The model under review builds one solid part; all positions refer to its coordinate system, in mm. A direction names the side the tool comes from. Give positions to 0.01 mm unless a question says otherwise; leave off trailing zeros. Loops run counter-clockwise (first coordinate to the right, second up) from the corner with the lowest first, then second, coordinate; pieces in that order, holes last. Notation, with made-up numbers: (-33.75, -25) - (-16.75, -25) arc R25 cw to (-16.75, -4) - close; hole circle Ø3 at (15, 37.25). An arc over 180 degrees is marked (long way). Return JSON: item names as keys, results as strings. Group by question number.
from build123d import *

# Parameters (mm, degrees)
SKETCH1_W                   = 12.7
SKETCH1_H                   = 483
BOSS_EXTRUDE1_DEPTH         = 3.175
EDGE_FLANGE1_DEPTH          = 12.7
TAP_DRILL_FOR_M4X0_7_TAP1_D = 3.3


# Sheet-metal steps are written as plain solids
with BuildPart() as part:
    # Sketch1 → Boss-Extrude1 (new body)
    with BuildSketch(Plane.XY):
        with Locations((6.35, 241.5)):
            Rectangle(SKETCH1_W, SKETCH1_H)
    extrude(amount=BOSS_EXTRUDE1_DEPTH)

    # Edge-Flange1 section (across the edge) → Edge-Flange1 (add)
    with BuildSketch(Plane(origin=(0, 493.5, 0), x_dir=(0, -1, 0), z_dir=(1, 0, 0))):
        with BuildLine():
            Line((-3.175, 10.5), (-3.175, 52.825))
            Line((-3.175, 52.825), (0, 52.825))
            Line((0, 52.825), (0, 10.5))
            ThreePointArc((0, 10.5), (3.075378798, 3.075378798), (10.5, 0))
            Line((10.5, 0), (10.5, -3.175))
            ThreePointArc((10.5, -3.175), (0.830314767, 0.830314767), (-3.175, 10.5))
        make_face()
    extrude(amount=EDGE_FLANGE1_DEPTH)

    # Tap Drill for M4x0.7 Tap1 (through all)
    with Locations(Plane.XY.offset(3.175)):
        with Locations((6.35, 10.5), (6.35, 31.5), (6.35, 52.5), (6.35, 73.5), (6.35, 94.5), (6.35, 115.5), (6.35, 136.5), (6.35, 157.5), (6.35, 178.5), (6.35, 199.5), (6.35, 220.5), (6.35, 241.5), (6.35, 262.5), (6.35, 283.5), (6.35, 304.5), (6.35, 325.5), (6.35, 346.5), (6.35, 367.5), (6.35, 388.5), (6.35, 409.5), (6.35, 430.5), (6.35, 451.5), (6.35, 472.5)):
            Hole(TAP_DRILL_FOR_M4X0_7_TAP1_D / 2)


solid = part.part
Item 1: For L1, parallel to X at y = 157, z = 1; L2, parallel to X at y = 241.5, z = 2.5; L3, parallel to Y at x = 2, z = -16.5 (3 decimals), list the stretches that pass through material, from the lowest coordinate up. Write a range as from..to.
Item 2: Take a section at B-B (y = 357). State the section outline as (x, z) points (3 decimals).
Item 3: Take a section at C-C (z = -25). State the section outline as (x, y) points (3 decimals).
Item 4: Tool access review of faces 1 (the face through (6, 493.5, -32)), 2 (the face through (0, 247, 2)): name each direction out of +Z, -Z, +X, -X, +Y, -Y from which nothing blocks a thin tool from reaching the whole face with its end or side.
Item 5: For P1, Ø1, axis at x = 6, z = -6, coming from the +Y side; P2, Ø4.5, axis at x = 6.35, y = 430.5, coming from the +Z side (3 decimals); P3, Ø5, axis at x = 6.5, y = 156, coming from the -Z side; P4, Ø5, axis at x = 11, z = -23.5, coming from the -Y side, all flat-tipped, find the tip position at first contact; note any pin that passes through.
Item 6: Take a section at A-A (x = 2.5). State the section outline as (y, z) points (3 decimals), then the cut area to 3 significant figures.
Check sheet entries:
{
 "1": {"L1": "x = 0..4.78, 7.92..12.7", "L2": "x = 0..4.7, 8..12.7", "L3": "y = 493.5..496.675"},
 "2": {"outline": "(0, 0) - (12.7, 0) - (12.7, 3.175) - (0, 3.175) - close"},
 "3": {"outline": "(0, 493.5) - (12.7, 493.5) - (12.7, 496.675) - (0, 496.675) - close"},
 "4": {"face 1": "-Z, +X, -X, -Y", "face 2": "+Z, -Z, -X, +Y, -Y"},
 "5": {"P1": "stops at y = 496.08", "P2": "stops at z = 3.175", "P3": "stops at z = 0", "P4": "stops at y = 493.5"},
 "6": {"outline": "(0, 0) - (483, 0) arc R10.5 cw to (493.5, -10.5) - (493.5, -52.825) - (496.675, -52.825) - (496.675, -10.5) arc R13.675 ccw to (483, 3.175) - (0, 3.175) - close", "area": "1,730 mm^2"}
}
